CAD build for the part. Positions are in the model's coordinates, mm. Face numbers are marked on the shaded views. A direction names the side the tool comes from. Coordinates: 2 decimals unless noted, no trailing zeros. Order: outer loops, then holes, each group sorted by start corner. A loop starts at its lowest first (then second) coordinate and runs counter-clockwise, first axis right, second up. Notation, with made-up numbers: (-9, 69) - (5, 69) arc R16 ccw to (5, 88) - close; hole circle Ø11 at (69.25, -8.5). An arc over 180 degrees is marked (long way). Write each question's results on one line, items separated by ' | '. Start each with the question number.
Q1. Band-saw the part on C-C, the plane y = -10.25. Write the cut outline in (x, z), then the cut area to 3 significant figures.
Q2. Which spindle directions (+Z, -Z, +X, -X, +Y, -Y) get a long thin tool onto all of the face, cutting with end or side? Do the marked faces 1, 2 and 3. Say none if no direction does.
Q3. Band-saw the part on B-B, the plane x = 16.5. Write the cut outline in (y, z), then the cut area to 3 significant figures.
Q4. Band-saw the part on A-A, the plane z = -14.25. Write the cut outline in (x, y), then the cut area to 3 significant figures.
Q5. Wall check: probe 1 along X at (y, z) = (-3.25, -8.5); probe 2 along X at (y, z) = (-10.75, -3); probe 3 along Y at (x, z) = (22, -14.5). Give the ranges that are in metal, low to high.
Q6. Pin check, flat tips, straight feed: P1, Ø6, axis at x = 19, z = -9, coming from the -Y side; P2, Ø2, axis at x = 30.5, z = -2.5, coming from the +Y side; P3, Ø2, axis at y = -2.5, z = -6, coming from the +X side. Stop position of each tip, or through.
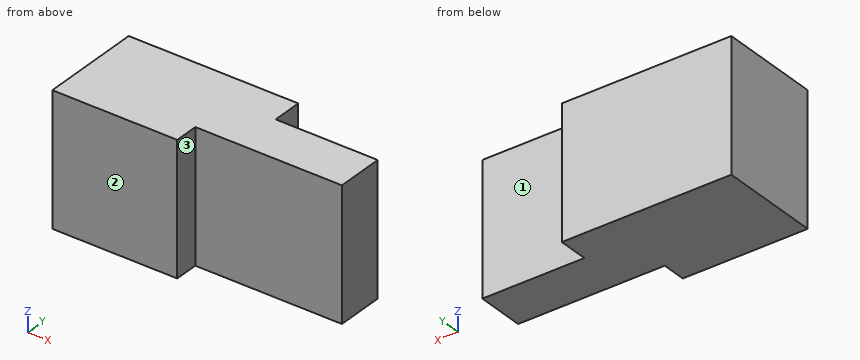
```python
from build123d import *

# Parameters (mm, degrees)
SKETCH1_W           = 33.8
SKETCH1_H           = 16.3
BOSS_EXTRUDE1_DEPTH = 12.7
SKETCH2_W           = 18.25
SKETCH2_H           = 3
SKETCH2_W_2         = 12.7
SKETCH2_H_2         = 3.75
CUT_EXTRUDE1_DEPTH  = 40.615905896


with BuildPart() as part:
    # Sketch1 → Boss-Extrude1 (new body)
    with BuildSketch(Plane(origin=(0, 0, 0), x_dir=(1, 0, 0), z_dir=(0, 1, 0))):
        with Locations((16.9, 8.15)):
            Rectangle(SKETCH1_W, SKETCH1_H)
    extrude(amount=-BOSS_EXTRUDE1_DEPTH)

    # Sketch2 → Cut-Extrude1 (cut, through all)
    with BuildSketch(Plane.XY):
        with Locations((24.675, -11.2)):
            Rectangle(SKETCH2_W, SKETCH2_H)
        with Locations((27.45, -1.875)):
            Rectangle(SKETCH2_W_2, SKETCH2_H_2)
    extrude(amount=-CUT_EXTRUDE1_DEPTH, mode=Mode.SUBTRACT)


solid = part.part
```
Results below:
1) outline: (0, -16.3) - (15.55, -16.3) - (15.55, 0) - (0, 0) - close | area: 253 mm²
2) face 1: +Z, -Z, +X, +Y | face 2: +Z, -Z, +X, -X, -Y | face 3: +Z, -Z, +X, -Y
3) outline: (-9.7, -16.3) - (0, -16.3) - (0, 0) - (-9.7, 0) - close | area: 158 mm²
4) outline: (0, -12.7) - (15.55, -12.7) - (15.55, -9.7) - (33.8, -9.7) - (33.8, -3.75) - (21.1, -3.75) - (21.1, 0) - (0, 0) - close | area: 327 mm²
5) probe 1: x = 0 to 21.1 | probe 2: x = 0 to 15.55 | probe 3: y = -9.7 to -3.75
6) P1: stops at y = -9.7 | P2: stops at y = -3.75 | P3: stops at x = 21.1
